from build123d import *

# Parameters (mm, degrees)
F1_DEPTH      = 101.6
F1_DEPTH_BACK = 101.6
F3_DEPTH      = 25.4
F5_DEPTH      = 25.4
F6_R          = 50.8


with BuildPart() as f1:
    # F0 (on Right) → F1 (new body, two sides)
    with BuildSketch(Plane.YZ) as f1_sk:
        with BuildLine():
            Line((50.8, -15.875), (0, -15.875))
            Line((0, -15.875), (-46.1643691758, -15.875))
            ThreePointArc((-46.1643691758, -15.875), (-56.6946528852, -19.05), (-67.2249365946, -15.875))
            Line((-67.2249365946, -15.875), (-254, -15.875))
            Line((-254, -15.875), (-254, -22.225))
            Line((-254, -22.225), (50.8, -22.225))
            Line((50.8, -22.225), (50.8, -15.875))
        make_face()
        with BuildLine():
            ThreePointArc((-67.2249365946, -15.875), (-56.6946528852, -19.05), (-46.1643691758, -15.875))
            Line((-46.1643691758, -15.875), (-56.6946528852, -15.875))
            Line((-56.6946528852, -15.875), (-67.2249365946, -15.875))
        make_face()
        with BuildLine():
            Line((-56.6946528852, -15.875), (-46.1643691758, -15.875))
            ThreePointArc((-46.1643691758, -15.875), (-39.9091769512, -9.0083460007), (-37.6446528852, 0))
            ThreePointArc((-37.6446528852, 0), (-65.7029988859, 16.785475934), (-67.2249365946, -15.875))
            Line((-67.2249365946, -15.875), (-56.6946528852, -15.875))
        make_face()
        with BuildLine():
            ThreePointArc((-40.8196528852, 0), (-45.4693327339, -11.2253201513), (-56.6946528852, -15.875))
            ThreePointArc((-56.6946528852, -15.875), (-67.9199730365, 11.2253201513), (-40.8196528852, 0))
        make_face(mode=Mode.SUBTRACT)
    extrude(amount=F1_DEPTH)
    extrude(f1_sk.sketch, amount=-F1_DEPTH_BACK)

    # F2 (on face) → F3 (cut)
    with BuildSketch(Plane.XY.offset(-15.875)):
        with BuildLine():
            Line((-101.6, -177.8), (-101.6, -254))
            Line((-101.6, -254), (-25.4, -254))
            ThreePointArc((-25.4, -254), (-79.2815367264, -231.6815367264), (-101.6, -177.8))
        make_face()
        with BuildLine():
            Line((101.6, -254), (101.6, -177.8))
            ThreePointArc((101.6, -177.8), (79.2815367264, -231.6815367264), (25.4, -254))
            Line((25.4, -254), (101.6, -254))
        make_face()
    extrude(amount=-F3_DEPTH, mode=Mode.SUBTRACT)

    # F4 (on face) → F5 (cut)
    with BuildSketch(Plane.XY.offset(-15.875)):
        with BuildLine():
            ThreePointArc((25.4, 9.525), (15.875, 0), (25.4, -9.525))
            Line((25.4, -9.525), (76.2, -9.525))
            ThreePointArc((76.2, -9.525), (85.725, 0), (76.2, 9.525))
            Line((76.2, 9.525), (25.4, 9.525))
        make_face()
        with BuildLine():
            Line((-76.2, -9.525), (-25.4, -9.525))
            ThreePointArc((-25.4, -9.525), (-18.6648079092, -6.7351920908), (-15.875, 0))
            ThreePointArc((-15.875, 0), (-18.6648079092, 6.7351920908), (-25.4, 9.525))
            Line((-25.4, 9.525), (-76.2, 9.525))
            ThreePointArc((-76.2, 9.525), (-85.725, 0), (-76.2, -9.525))
        make_face()
        with BuildLine():
            Line((-25.4, -89.789), (-76.2, -89.789))
            ThreePointArc((-76.2, -89.789), (-85.725, -99.314), (-76.2, -108.839))
            Line((-76.2, -108.839), (-25.4, -108.839))
            ThreePointArc((-25.4, -108.839), (-15.875, -99.314), (-25.4, -89.789))
        make_face()
        with BuildLine():
            Line((-25.4, -138.303), (-76.2, -138.303))
            ThreePointArc((-76.2, -138.303), (-85.725, -147.828), (-76.2, -157.353))
            Line((-76.2, -157.353), (-25.4, -157.353))
            ThreePointArc((-25.4, -157.353), (-15.875, -147.828), (-25.4, -138.303))
        make_face()
        with BuildLine():
            Line((-25.4, -186.817), (-76.2, -186.817))
            ThreePointArc((-76.2, -186.817), (-85.725, -196.342), (-76.2, -205.867))
            Line((-76.2, -205.867), (-25.4, -205.867))
            ThreePointArc((-25.4, -205.867), (-15.875, -196.342), (-25.4, -186.817))
        make_face()
        with BuildLine():
            ThreePointArc((25.4, -186.817), (15.875, -196.342), (25.4, -205.867))
            Line((25.4, -205.867), (76.2, -205.867))
            ThreePointArc((76.2, -205.867), (85.725, -196.342), (76.2, -186.817))
            Line((76.2, -186.817), (25.4, -186.817))
        make_face()
        with BuildLine():
            ThreePointArc((25.4, -138.303), (15.875, -147.828), (25.4, -157.353))
            Line((25.4, -157.353), (76.2, -157.353))
            ThreePointArc((76.2, -157.353), (85.725, -147.828), (76.2, -138.303))
            Line((76.2, -138.303), (25.4, -138.303))
        make_face()
        with BuildLine():
            ThreePointArc((76.2, -108.839), (85.725, -99.314), (76.2, -89.789))
            Line((76.2, -89.789), (25.4, -89.789))
            ThreePointArc((25.4, -89.789), (15.875, -99.314), (25.4, -108.839))
            Line((25.4, -108.839), (76.2, -108.839))
        make_face()
    extrude(amount=-F5_DEPTH, mode=Mode.SUBTRACT)

    # F6
    f6_edges = [f1.edges().sort_by_distance(p)[0] for p in [
        (101.6, 50.8, -19.05),
        (-101.6, 50.8, -19.05),
    ]]
    fillet(f6_edges, radius=F6_R)


solid = f1.part
Can you work these out from the model? Positions are in its coordinate system, mm. A direction names the side the tool comes from. Give positions to 0.01 mm unless a question says otherwise; leave off trailing zeros. Loops run counter-clockwise (first coordinate to the right, second up) from the corner with the lowest first, then second, coordinate; pieces in that order, holes last. Notation, with made-up numbers: (-2, 13.25) -> (27, 13.25) arc R31 cw to (27, 37.25) -> close; hole circle Ø10 at (66, 9). An arc over 180 degrees is marked (long way). Return JSON: item names as keys, results as strings.
Q1. We'd pull the mould along X, two halves only. Please class faces 3 (the face through (-78.686, -232.271, -19.006)), 4 (the face through (79.871, -231.086, -19.006)), 5 (the face through (-85.723, -196.133, -19.006)): released by +X, released by -X, zero draft, split by the parting line, or undercut.
Checks:
{"face 3": "released by -X", "face 4": "released by +X", "face 5": "undercut"}
Q2. On a 3-axis mill with a long thin cutter (end or side, diameter ignored), from which of +Z, -Z, +X, -X, +Y, -Y can I reach the whole of each face in a straight line? I mean faces 1 (the face through (86.324, 36.314, -19.006)), 2 (the face through (-15.877, -196.551, -19.006)). Say none if no direction works.
Checks:
{"face 1": "+Z, -Z, +X, +Y", "face 2": "+Z, -Z"}
Q3. I want a section at D-D, the plane z = -12.5. List the corners of the cut face in (x, y) for me.
Checks:
{"outline": "(-101.6, -71.07) -> (101.6, -71.07) -> (101.6, -66.48) -> (-101.6, -66.48) -> close; (-101.6, -46.91) -> (101.6, -46.91) -> (101.6, -42.32) -> (-101.6, -42.32) -> close"}
Q4. I want a section at C-C, the plane x = -72. List the corners of the cut face in (y, z) for me (3 decimals).
Checks:
{"outline": "(-238.09, -22.225) -> (-205.867, -22.225) -> (-205.867, -15.875) -> (-238.09, -15.875) -> close; (-186.817, -22.225) -> (-157.353, -22.225) -> (-157.353, -15.875) -> (-186.817, -15.875) -> close; (-138.303, -22.225) -> (-108.839, -22.225) -> (-108.839, -15.875) -> (-138.303, -15.875) -> close; (-89.789, -22.225) -> (-9.525, -22.225) -> (-9.525, -15.875) -> (-46.164, -15.875) arc R19.05 ccw (long way) to (-67.225, -15.875) -> (-89.789, -15.875) -> close; (9.525, -22.225) -> (46.165, -22.225) -> (46.165, -15.875) -> (9.525, -15.875) -> close; hole circle Ø31.75 at (-56.695, 0)"}
Q5. I need wall thicknesses on probe 1 along Z at (x, y) = (-91, -42.5) (3 decimals); probe 2 along Y at (x, z) = (65, 0); probe 3 along Z at (x, y) = (-43.5, -237.5) (3 decimals). Which ranges of each line are inside material? Lowest first, please.
Checks:
{"probe 1": "z = -22.225 to -15.875, -12.705 to -7.108, 7.108 to 12.705", "probe 2": "y = -75.74 to -72.57, -40.82 to -37.64", "probe 3": "z = -22.225 to -15.875"}
Q6. For pin 1 Ø1.9 at (x, z) = (51, -18.5) entering from -Y; pin 2 Ø10 at (x, z) = (-31.5, 4.5) entering from +Y; pin 3 Ø1.9 at (x, z) = (63, -19.5) entering from +Y, each with a flat end and sliding along its axis, tell me the tip position at first contact or that it passes through.
Checks:
{"pin 1": "stops at y = -249.9", "pin 2": "stops at y = -37.64", "pin 3": "stops at y = 49.54"}
Q7. I want a section at A-A, the plane x = 41. List the corners of the cut face in (y, z) for me (3 decimals).
Checks:
{"outline": "(-252.386, -22.225) -> (-205.867, -22.225) -> (-205.867, -15.875) -> (-252.386, -15.875) -> close; (-186.817, -22.225) -> (-157.353, -22.225) -> (-157.353, -15.875) -> (-186.817, -15.875) -> close; (-138.303, -22.225) -> (-108.839, -22.225) -> (-108.839, -15.875) -> (-138.303, -15.875) -> close; (-89.789, -22.225) -> (-9.525, -22.225) -> (-9.525, -15.875) -> (-46.164, -15.875) arc R19.05 ccw (long way) to (-67.225, -15.875) -> (-89.789, -15.875) -> close; (9.525, -22.225) -> (50.8, -22.225) -> (50.8, -15.875) -> (9.525, -15.875) -> close; hole circle Ø31.75 at (-56.695, 0)"}
Q8. I want a section at B-B, the plane y = -152.5. List the corners of the cut face in (x, z) for me (3 decimals), then the cut area to 3 significant figures.
Checks:
{"outline": "(-101.6, -22.225) -> (-84.5, -22.225) -> (-84.5, -15.875) -> (-101.6, -15.875) -> close; (-17.1, -22.225) -> (17.1, -22.225) -> (17.1, -15.875) -> (-17.1, -15.875) -> close; (84.5, -22.225) -> (101.6, -22.225) -> (101.6, -15.875) -> (84.5, -15.875) -> close", "area": "434 mm2"}
